Autodesk Inventor part; units mm, degrees
ref_plane "YZ Plane" through (0, 0, 0) normal (1, 0, 0) x (0, 1, 0)
ref_plane "XZ Plane" through (0, 0, 0) normal (0, 1, 0) x (-1, 0, 0)
ref_plane "XY Plane" through (0, 0, 0) normal (0, 0, 1) x (1, 0, 0)
sketch "スケッチ1" plane through (0, 0, 0) normal (0, 1, 0) x (-1, 0, 0)
  line L0 (0, 0) -> (-9, 0)
  line L1 (-9, 0) -> (-9, 9)
  line L2 (-9, 9) -> (0, 9)
  line L3 (0, 9) -> (0, 0)
  line L4 (-1.2, 7.8) -> (-7.8, 7.8)
  line L5 (-7.8, 7.8) -> (-7.8, 1.2)
  line L6 (-7.8, 1.2) -> (-1.2, 1.2)
  line L7 (-1.2, 1.2) -> (-1.2, 7.8)
  dimension "d0" = 9
  dimension "d1" = 9
  dimension "d2" = 6.6
  dimension "d3" = 6.6
  dimension "d4" = 1.2
  dimension "d5" = 1.2
extrude "押し出し1" add sketch "スケッチ1" along normal blind 58.5
sketch "スケッチ2" plane through (0, 0, 9) normal (0, 0, 1) x (1, 0, 0)
  line L0 (0, 58.5) -> (9, 58.5)
  line L1 (9, 0) -> (9, 58.5)
  line L2 (0, 0) -> (9, 0)
  point P0 (4.5, 4.5)
  point P1 (4.5, 54)
  dimension "d8" = 4.5
  dimension "d9" = 4.5
  dimension "d10" = 4.5
  dimension "d11" = 4.5
hole "穴1" at (4.5, 4.5, 9) at (4.5, 54, 9) direction (0, 0, -1) diameter 3 end through all
sketch "スケッチ3" plane through (9, 0, 9) normal (1, 0, 0) x (0, 0, -1)
  line L0 (0, 0) -> (9, 0)
  line L1 (0, 0) -> (0, 58.5)
  line L2 (0, 58.5) -> (9, 58.5)
  point P0 (4.5, 13.5)
  point P1 (4.5, 39.5)
  dimension "d19" = 13.5
  dimension "d20" = 4.5
  dimension "d21" = 19
  dimension "d22" = 4.5
hole "穴2" at (9, 13.5, 4.5) at (9, 39.5, 4.5) direction (-1, 0, 0) diameter 3 end through all
sketch "スケッチ4" plane through (0, 0, 0) normal (-1, 0, 0) x (0, 0, 1)
  line L0 (9, 0) -> (0, 0)
  line L1 (4.5, 0) -> (4.5, 58.5)
  line L2 (1.2, 58.5) -> (7.8, 58.5)
  line L3 (0, 0) -> (0, 58.5)
  circle A0 centre (4.5, 13.5) radius 1.5
  circle A1 centre (4.5, 39.5) radius 1.5
  point P0 (4.5, 6.75)
  point P1 (4.5, 20)
  point P2 (4.5, 33)
  point P3 (4.5, 45.8333)
  point P4 (4.5, 52.1667)
  point P5 (4.5, 26.5)
  dimension "d30" = 4.5
  dimension "d31" = 13.5
  dimension "d32" = 6.75
  dimension "d33" = 26
  dimension "d34" = 6.5
  dimension "d35" = 6.5
  dimension "d36" = 6.5
  dimension "d37" = 19
  dimension "d38" = 6.3333
  dimension "d39" = 6.3333
hole "穴3" at (0, 6.75, 4.5) at (0, 20, 4.5) at (0, 33, 4.5) at (0, 45.8333, 4.5) at (0, 52.1667, 4.5) at (0, 26.5, 4.5) direction (1, 0, 0) diameter 5 end through all
sketch "スケッチ5" plane through (9, 0, 0) normal (0, 0, -1) x (-1, 0, 0)
  circle A0 centre (4.5, 4.5) radius 1.5
  circle A1 centre (4.5, 54) radius 1.5
  line L0 (4.5, 4.5) -> (4.5, 54)
  point P0 (9, 0)
  point P1 (4.5, 10.6875)
  point P2 (4.5, 16.875)
  point P3 (4.5, 23.0625)
  point P4 (4.5, 29.25)
  point P5 (4.5, 35.4375)
  point P6 (4.5, 41.625)
  point P7 (4.5, 47.8125)
  dimension "d47" = 49.5
  dimension "d48" = 6.1875
  dimension "d51" = 6.1875
hole "穴4" at (4.5, 10.6875, 0) at (4.5, 16.875, 0) at (4.5, 23.0625, 0) at (4.5, 29.25, 0) at (4.5, 35.4375, 0) at (4.5, 41.625, 0) at (4.5, 47.8125, 0) direction (0, 0, 1) diameter 5 end through all
equation "\"d5\" = d4"
properties part number "上下直動9x9_4" material "アルミニウム 6061"
The model under review builds one solid part; all positions refer to its coordinate system, in mm. A direction names the side the tool comes from. Coordinates: 2 decimals unless noted, no trailing zeros. Loops run counter-clockwise (first coordinate to the right, second up) from the corner with the lowest first, then second, coordinate; pieces in that order, holes last. Notation, with made-up numbers: (36, -2.75) -> (54, -2.75) arc R16 cw to (54, 1.25) -> close; hole circle Ø6 at (39.25, 33.25). An arc over 180 degrees is marked (long way). Use a Markdown table: item, result. Add a question column.
1. To check wall thickness, follow line 1 (Z direction, x = 7.5, y = 25.5); line 2 (Z direction, x = 8.7, y = 20). State the ranges of each line that lie inside material, in increasing order.
2. Add section A-A on x = 4.5. Give the number of separate pieces and of enclosed holes in the cut face, plus the area to 3 significant figures.
3. Add section D-D on y = 5.5. Write out the cut boundary in (x, z), plus the area to 3 significant figures.
4. Add section B-B on y = 54. Write out the cut boundary in (x, z).
5. Machinability: for faces 4 (the face through (7.8, 29, 6)), 5 (the face through (0.592, 40.964, 4.825)), which of the approach directions +Z, -Z, +X, -X, +Y, -Y give a long, thin tool a straight path to every point of the face, cutting with its end or side? Answer none if there is none.
6. Draft analysis for pull direction X (two halves, no side actions). For faces 1 (the face through (5.4, 55.2, 8.4)), 2 (the face through (9, 29, 3)), 3 (the face through (8.4, 43.7, 5.8)), state which applies: pulls with the +X half, pulls with the -X half, needs draft (parallel to the pull), parting line crosses it, or undercut.
Returned:
| question | item | result |
|---|---|---|
| 1 | line 1 | z = 0 to 1.2, 7.8 to 9 |
| 1 | line 2 | z = 0 to 2, 7 to 9 |
| 2 | separate pieces | 20 |
| 2 | enclosed holes | 0 |
| 2 | area | 42.0 mm² |
| 3 | outline | (0, 0) -> (3.38, 0) -> (3.38, 1.2) -> (1.2, 1.2) -> (1.2, 2.33) -> (0, 2.33) -> close; (0, 6.67) -> (1.2, 6.67) -> (1.2, 7.8) -> (3.38, 7.8) -> (3.38, 9) -> (0, 9) -> close; (5.62, 0) -> (9, 0) -> (9, 2.33) -> (7.8, 2.33) -> (7.8, 1.2) -> (5.62, 1.2) -> close; (5.62, 7.8) -> (7.8, 7.8) -> (7.8, 6.67) -> (9, 6.67) -> (9, 9) -> (5.62, 9) -> close |
| 3 | area | 21.7 mm² |
| 4 | outline | (0, 0) -> (3, 0) -> (3, 1.2) -> (1.2, 1.2) -> (1.2, 2.8) -> (0, 2.8) -> close; (0, 6.2) -> (1.2, 6.2) -> (1.2, 7.8) -> (3, 7.8) -> (3, 9) -> (0, 9) -> close; (6, 0) -> (9, 0) -> (9, 2.8) -> (7.8, 2.8) -> (7.8, 1.2) -> (6, 1.2) -> close; (6, 7.8) -> (7.8, 7.8) -> (7.8, 6.2) -> (9, 6.2) -> (9, 9) -> (6, 9) -> close |
| 5 | face 4 | +Y, -Y |
| 5 | face 5 | +X, -X |
| 6 | face 1 | undercut |
| 6 | face 2 | pulls with the +X half |
| 6 | face 3 | needs draft |
